Model file for the job. Use its own axes, mm. A direction names the side the tool comes from. Round coordinates to 2 decimals unless told otherwise and drop trailing zeros. Loops run counter-clockwise (first coordinate to the right, second up) from the corner with the lowest first, then second, coordinate; pieces in that order, holes last. Notation, with made-up numbers: M 20,79.25 L 38,79.25 A15 ccw 38,96.25 Z; hole C -7.5,-35 d10. An arc over 180 degrees is marked long. Answer in a Markdown table with one row per item.
from build123d import *

# Parameters (mm, degrees)
ENL_V_START             = -2
ENL_V_MAT_EXTRU_1_DEPTH = 1.3


with BuildPart() as part:
    # Esquisse1 → Révolution1 (revolve)
    with BuildSketch(Plane.XY, mode=Mode.PRIVATE) as r_volution1_sk:
        Polygon((0, -2), (2.5, -2), (2.5, 0), (2.3, 0), (1.49, 0), (1.49, 6), (1.2, 6), (1.2, 6.5), (1.45, 6.5), (1.45, 9.7), (1.15, 10), (0, 10), align=None)
    revolve(r_volution1_sk.sketch.rotate(Axis((0, -4, 0), (0, 1, 0)), 90), axis=Axis((0, -4, 0), (0, 1, 0)))

    # Esquisse2 → Enlèv. mat.-Extru.1 (cut)
    with BuildSketch(Plane(origin=(0, 0, 0), x_dir=(1, 0, 0), z_dir=(0, 1, 0)).offset(ENL_V_START)):
        Polygon((1.154700538, 0), (0.577350269, 1), (-0.577350269, 1), (-1.154700538, 0), (-0.577350269, -1), (0.577350269, -1), align=None)
    extrude(amount=ENL_V_MAT_EXTRU_1_DEPTH, mode=Mode.SUBTRACT)


solid = part.part
1. Saw through at A-A (x = 0). Write the cut outline in (y, z), and give its area (3 significant figures).
Verdict:
| item | result |
|---|---|
| outline | M -2,-2.5 L 0,-2.5 L 0,-1.49 L 6,-1.49 L 6,-1.2 L 6.5,-1.2 L 6.5,-1.45 L 9.7,-1.45 L 10,-1.15 L 10,1.15 L 9.7,1.45 L 6.5,1.45 L 6.5,1.2 L 6,1.2 L 6,1.49 L 0,1.49 L 0,2.5 L -2,2.5 L -2,1 L -0.7,1 L -0.7,-1 L -2,-1 Z |
| area | 36.5 mm² |
2. Saw through at B-B (y = 4). Write the cut outline in (x, z).
Verdict:
| item | result |
|---|---|
| outline | C 0,0 d2.98 |
3. Saw through at C-C (z = 1.9). Write the cut outline in (x, y).
Verdict:
| item | result |
|---|---|
| outline | M -1.62,-2 L 1.62,-2 L 1.62,0 L -1.62,0 Z |
4. Tool access for faces 4 (the flat face through (0, -1, -1)), 5 (the flat face through (0, 10, 0)), 6 (the cylindrical face through (-0.06, 8.12, 1.45)): list every direction of +Z, -Z, +X, -X, +Y, -Y with a clear straight run to the whole face (end or side of a thin tool).
Verdict:
| item | result |
|---|---|
| face 4 | -Y |
| face 5 | +Z, -Z, +X, -X, +Y |
| face 6 | +Y |
5. Pin check, flat tips, straight feed: pin 1 (0.6 mm diameter, centred on x = 0, z = 0, fed in from -Y); pin 2 (0.6 mm diameter, centred on x = -0.5, y = -1, fed in from -Z); pin 3 (1.5 mm diameter, centred on y = 2.5, z = 0.5, fed in from -X). Stop position of each tip, or through.
Verdict:
| item | result |
|---|---|
| pin 1 | stops at y = -0.7 |
| pin 2 | stops at z = -2.49 |
| pin 3 | stops at x = -1.49 |
6. Wall check: probe 1 along Y at (x, z) = (-0.45, 0.1); probe 2 along Y at (x, z) = (-1.95, 0.3); probe 3 along Z at (x, y) = (0.7, -1). Give the ranges that are in metal, low to high.
Verdict:
| item | result |
|---|---|
| probe 1 | y = -0.7 to 10 |
| probe 2 | y = -2 to 0 |
| probe 3 | z = -2.4 to -0.79, 0.79 to 2.4 |
7. Mould opens along Z. For faces 1 (the flat face through (1, -2, 1)), 2 (the flat face through (-0.87, -1.36, 0.49)), 3 (the cylindrical face through (-1.01, 6.25, -0.65)) say: +Z half, -Z half, draft (parallel to the pull), parting line (faces both ways), or undercut.
Verdict:
| item | result |
|---|---|
| face 1 | draft |
| face 2 | undercut |
| face 3 | parting line |
